Part model, mm, in its own coordinate system. Face numbers are marked on the shaded views. A direction names the side the tool comes from. Round coordinates to 2 decimals unless told otherwise and drop trailing zeros. Loops run counter-clockwise (first coordinate to the right, second up) from the corner with the lowest first, then second, coordinate; pieces in that order, holes last. Notation, with made-up numbers: (30, 57) -> (40, 57) arc R26 ccw to (40, 78) -> close; hole circle Ø6 at (24.5, 77). An arc over 180 degrees is marked (long way). Answer as CSV lines item,"result".
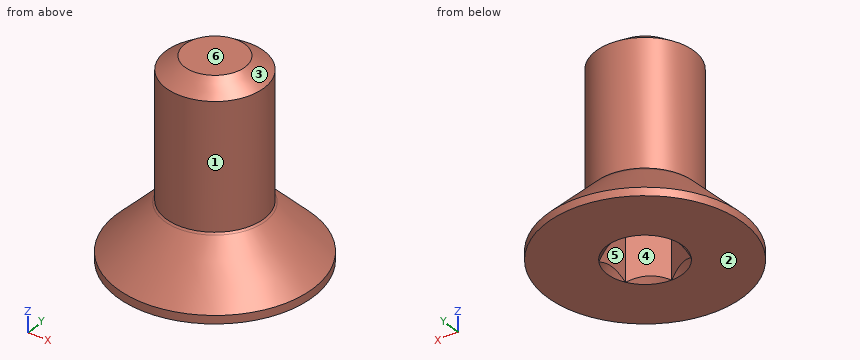
from build123d import *

# Parameters (mm, degrees)
SKETCH1_R          = 1.5
EXTRUDE1_DEPTH     = 6
SKETCH6_R          = 3
EXTRUDE2_DEPTH     = 1.7
CUT_EXTRUDE1_DEPTH = 1.5
SKETCH8_R          = 1.154700538
CUT_EXTRUDE2_DEPTH = 7
CUT_EXTRUDE2_TAPER = 45


with BuildPart() as part:
    # Sketch1 → Extrude1 (new body)
    with BuildSketch(Plane.XY):
        Circle(SKETCH1_R)
    extrude(amount=-EXTRUDE1_DEPTH)

    # Sketch4 → Cut-Revolve1 (revolve, cut)
    with BuildSketch(Plane(origin=(0, 0, 0), x_dir=(0, 0, -1), z_dir=(1, 0, 0)), mode=Mode.PRIVATE) as cut_revolve1_sk:
        Polygon((0.405251783, 1.5), (0, 0.921240474), (0, 1.5), align=None)
    revolve(cut_revolve1_sk.sketch.rotate(Axis((0, 0, 0), (0, 0, -1)), 90), axis=Axis((0, 0, 0), (0, 0, -1)), mode=Mode.SUBTRACT)  # turned: the seam where the file's is

    # Sketch6 → Extrude2 (add)
    with BuildSketch(Plane(origin=(0, 0, -6), x_dir=(-1, 0, 0), z_dir=(0, 0, -1))):
        Circle(SKETCH6_R)
    extrude(amount=-EXTRUDE2_DEPTH)

    # Sketch10 → Cut-Revolve2 (revolve, cut)
    with BuildSketch(Plane(origin=(0, 0, 0), x_dir=(0, 0, -1), z_dir=(1, 0, 0)), mode=Mode.PRIVATE) as cut_revolve2_sk:
        Polygon((5.75, -3), (4.3, -1.55), (4.3, -3), align=None)
    revolve(cut_revolve2_sk.sketch.rotate(Axis((0, 0, 0), (0, 0, -1)), 270), axis=Axis((0, 0, 0), (0, 0, -1)), mode=Mode.SUBTRACT)  # turned: the seam where the file's is

    # Sketch11 → Revolve1 (revolve)
    with BuildSketch(Plane(origin=(0, 0, 0), x_dir=(0, 0, -1), z_dir=(1, 0, 0)), mode=Mode.PRIVATE) as revolve1_sk:
        with BuildLine():
            Line((3.395250469, 1.175240474), (3.395250469, 0))
            Line((3.395250469, 0), (4.3, 0))
            Line((4.3, 0), (4.3, 1.55))
            ThreePointArc((4.3, 1.55), (3.884897387, 1.272637301), (3.395250469, 1.175240474))
        make_face()
    revolve(revolve1_sk.sketch.rotate(Axis((0, 0, 0), (0, 0, -1)), 90), axis=Axis((0, 0, 0), (0, 0, -1)))  # turned: the seam where the file's is

    # Sketch7 → Cut-Extrude1 (cut)
    with BuildSketch(Plane.XY.offset(-6)):
        Polygon((0, 1.154700538), (-1, 0.577350269), (-1, -0.577350269), (0, -1.154700538), (1, -0.577350269), (1, 0.577350269), align=None)
    extrude(amount=CUT_EXTRUDE1_DEPTH, mode=Mode.SUBTRACT)

    # Sketch8 → Cut-Extrude2 (cut, through all)
    with BuildSketch(Plane.XY.offset(-6)):
        Circle(SKETCH8_R)
    extrude(amount=CUT_EXTRUDE2_DEPTH, taper=CUT_EXTRUDE2_TAPER, mode=Mode.SUBTRACT)


solid = part.part
Q1. Which spindle directions (+Z, -Z, +X, -X, +Y, -Y) get a long thin tool onto all of the face, cutting with end or side? Do the marked faces 1 and 2. Say none if no direction does.
Geometry results:
face 1,"+Z"
face 2,"-Z, +X, -X, +Y, -Y"
Q2. Two-plate mould, pull along Y, no slides. Class the marked faces 3, 4, 5 and 6: pulls with the +Y half, pulls with the -Y half, needs draft (parallel to the pull), parting line crosses it, or undercut.
Geometry results:
face 3,"parting line crosses it"
face 4,"undercut"
face 5,"undercut"
face 6,"needs draft"
Q3. Drop flat-ended pins along their axis: P1, Ø2, axis at y = 2, z = -4, coming from the -X side; P2, Ø3, axis at x = 0.5, z = -3.5, coming from the +Y side; P3, Ø0.6, axis at x = 0, y = 0.5, coming from the -Z side. Give the stop position or say it passes through.
Geometry results:
P1,"x = -1.5"
P2,"y = 2.22"
P3,"z = -4.5"
Q4. Drill centre lines: line 1 along Y through (x, z) = (0.4, -4.8); line 2 along Y through (x, z) = (-0.65, -5.2); line 3 along Z through (x, y) = (0.3, 2.1). Where is each one in solid material? Low to high.
Geometry results:
line 1,"-2.01 to -0.92, 0.92 to 2.01"
line 2,"-2.36 to -0.78, 0.78 to 2.36"
line 3,"-6 to -4.87"
Q5. Saw through at C-C, the plane z = -4.1. Write the cut outline in (x, y).
Geometry results:
outline,"circle Ø3 at (0, 0)"
Q6. Saw through at A-A, the plane z = -5.4. Write the cut outline in (x, y), then the cut area to 3 significant figures.
Geometry results:
outline,"circle Ø5.3 at (0, 0); hole (-1, -0.58) -> (0, -1.15) -> (1, -0.58) -> (1, 0.58) -> (0, 1.15) -> (-1, 0.58) -> close"
area,"18.6 mm2"
Q7. Saw through at B-B, the plane y = 0. Write the cut outline in (x, z), then the cut area to 3 significant figures.
Geometry results:
outline,"(-3, -6) -> (-1.15, -6) -> (-1, -5.85) -> (-1, -4.5) -> (1, -4.5) -> (1, -5.85) -> (1.15, -6) -> (3, -6) -> (3, -5.75) -> (1.55, -4.3) arc R1.28 cw to (1.5, -4.25) -> (1.5, -0.41) -> (0.92, 0) -> (-0.92, 0) -> (-1.5, -0.41) -> (-1.5, -4.25) arc R1.28 cw to (-1.55, -4.3) -> (-3, -5.75) -> close"
area,"17.7 mm2"
